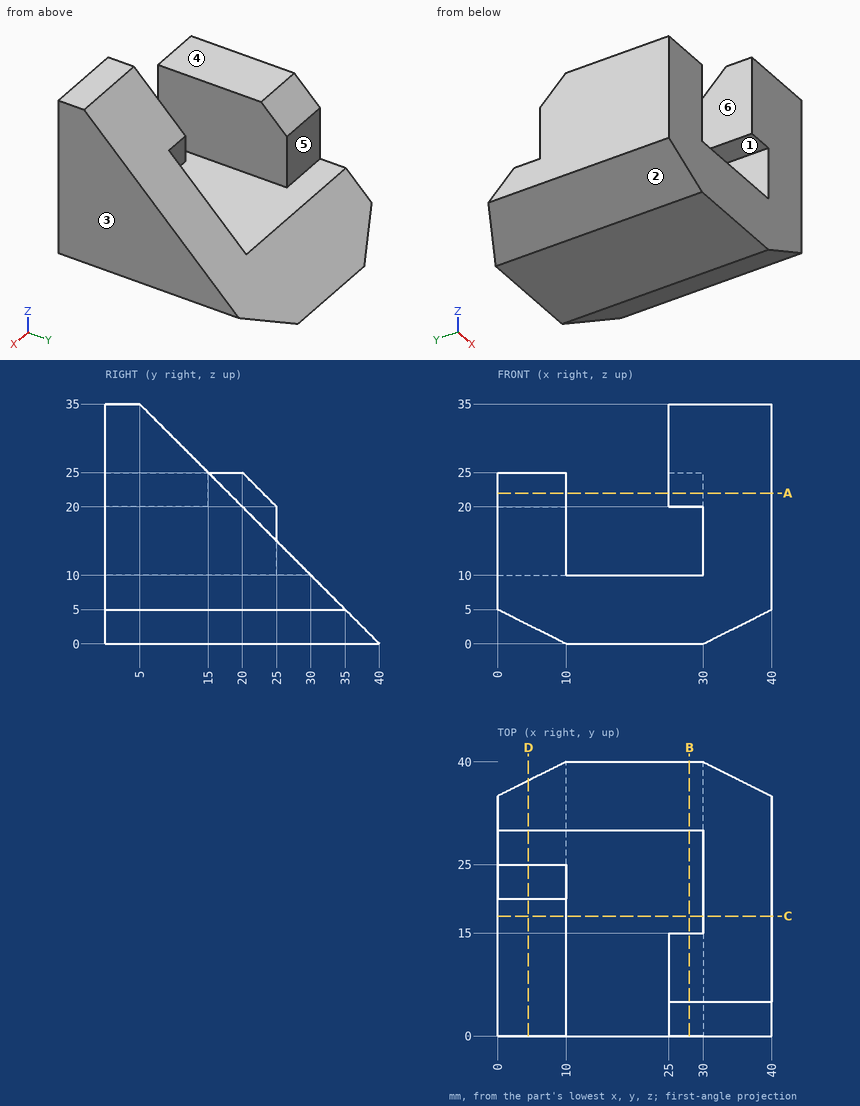
Study the drawing (mm; zero at the part's minimum x, y, z) and answer. A direction names the side the tool comes from. Coordinates: 2 decimals unless noted, no trailing zeros. Write each loop counter-clockwise with the first axis right and the second up, starting at its lowest first coordinate (ties: lowest second). Pieces come first, ordered by that corner, then holes. Notation, with made-up numbers: (-21.75, 56.25) -> (17.25, 56.25) arc R21 ccw to (17.25, 83.25) -> close; hole circle Ø6 at (81.5, -9). An arc over 180 degrees is marked (long way). Write item = value, one per line.
(1) Section D-D on x = 4.5 is taken. Write down the section's boundary in (y, z), plus the area to 3 significant figures.
From the geometry:
outline = (0, 2.75) -> (37.25, 2.75) -> (30, 10) -> (25, 10) -> (25, 20) -> (20, 25) -> (0, 25) -> close
area = 606 mm2
(2) Section A-A on z = 22 is taken. Write down the section's boundary in (x, y).
From the geometry:
outline = (0, 0) -> (10, 0) -> (10, 23) -> (0, 23) -> close; (25, 0) -> (40, 0) -> (40, 18) -> (30, 18) -> (30, 15) -> (25, 15) -> close
(3) Straight lines are drawn through the part: L1, parallel to X at y = 10, z = 14; L2, parallel to X at y = 8, z = 31; L3, parallel to X at y = 5, z = 20.5. For each, find the intervals that lie inside material, in ascending order. Write a range as from..to.
From the geometry:
L1 = 0..10, 30..40
L2 = 25..40
L3 = 0..10, 25..40
(4) For a pull along Z with two mould halves and no side action, classify the marked faces 1, 2 and 3 as +Z half, -Z half, draft (parallel to the pull), parting line (faces both ways), or undercut.
From the geometry:
face_1 = undercut
face_2 = -Z half
face_3 = draft
(5) Section B-B on x = 28 is taken. Write down the section's boundary in (y, z), plus the area to 3 significant figures.
From the geometry:
outline = (0, 0) -> (40, 0) -> (30, 10) -> (0, 10) -> close; (0, 20) -> (15, 20) -> (15, 25) -> (5, 35) -> (0, 35) -> close
area = 525 mm2
(6) Which of the six approach directions +Z, -Z, +X, -X, +Y, -Y give full straight-line access (tool end or side, diameter ignored) to the marked faces 4, 5 and 6?
From the geometry:
face_4 = +Z, -X, +Y, -Y
face_5 = +Z, -X, +Y
face_6 = +Z, +Y, -Y
(7) Given pin 1 Ø8 at (x, y) = (18, 20.5) entering from +Z; pin 2 Ø8 at (y, z) = (10, 25.5) entering from -X; pin 3 Ø6 at (y, z) = (13, 30.5) entering from -X; pin 4 Ø3 at (x, y) = (7, 15) entering from +Z, each flat-ended and moving along its own axis, determine where each tip first touches the part or whether it passes through.
From the geometry:
pin_1 = 10
pin_2 = 0
pin_3 = 25
pin_4 = 25
(8) Section C-C on y = 17.5 is taken. Write down the section's boundary in (x, z).
From the geometry:
outline = (0, 5) -> (10, 0) -> (30, 0) -> (40, 5) -> (40, 22.5) -> (30, 22.5) -> (30, 10) -> (10, 10) -> (10, 25) -> (0, 25) -> close
